Part model, mm, in its own coordinate system. Face numbers are marked on the shaded views. A direction names the side the tool comes from. Round coordinates to 2 decimals unless told otherwise and drop trailing zeros. Loops run counter-clockwise (first coordinate to the right, second up) from the corner with the lowest first, then second, coordinate; pieces in that order, holes last. Notation, with made-up numbers: (16, -8.75) -> (30, -8.75) arc R11 ccw to (30, 9.25) -> close; hole circle Ø11 at (-9, 79). An arc over 180 degrees is marked (long way). Answer as CSV lines item,"result".
from build123d import *

# Parameters (mm, degrees)
EXTRUDE_THIN1_DEPTH        = 36
CONVERT_SOLID1_START       = -36
CONVERT_SOLID1_DEPTH       = 72
CONVERT_SOLID1_2_DEPTH     = 72
F_6_5_6_5_DIAMETER_HOLE1_D = 6.5
F_6_5_6_5_DIAMETER_HOLE2_D = 6.5


# Read off the part's stored shape, not the designer's step: Convert-Solid1
with BuildPart() as part:
    # Sketch1 → Extrude-Thin1 (new, symmetric)
    with BuildSketch(Plane.XY):
        Polygon((-50, -56), (-50, 0), (50, 0), (50, -56), (46, -56), (46, -4), (-46, -4), (-46, -56), align=None)
    extrude(amount=EXTRUDE_THIN1_DEPTH, both=True)

    # Convert-Solid1 outline → Convert-Solid1 (cut)
    with BuildSketch(Plane.XY.offset(CONVERT_SOLID1_START)):
        with BuildLine():
            Line((50, 0), (44, 0))
            ThreePointArc((44, 0), (48.242640687, -1.757359313), (50, -6))
            Line((50, -6), (50, 0))
        make_face()
        with BuildLine():
            ThreePointArc((-50, -6), (-48.242640687, -1.757359313), (-44, 0))
            Line((-44, 0), (-50, 0))
            Line((-50, 0), (-50, -6))
        make_face()
    extrude(amount=CONVERT_SOLID1_DEPTH, mode=Mode.SUBTRACT)

    # Convert-Solid1 2 outline → Convert-Solid1 2 (add)
    with BuildSketch(Plane.XY.offset(CONVERT_SOLID1_START)):
        with BuildLine():
            Line((46, -4), (44, -4))
            ThreePointArc((44, -4), (45.414213562, -4.585786438), (46, -6))
            Line((46, -6), (46, -4))
        make_face()
        with BuildLine():
            ThreePointArc((-46, -6), (-45.414213562, -4.585786438), (-44, -4))
            Line((-44, -4), (-46, -4))
            Line((-46, -4), (-46, -6))
        make_face()
    extrude(amount=CONVERT_SOLID1_2_DEPTH)

    # Ø6.5 (6.5) Diameter Hole1 (through all)
    with Locations(Plane(origin=(-92.5, 4, 244.5), x_dir=(1, 0, 0), z_dir=(0, 1, 0))):
        with Locations((-122.5, 244.5), (-62.5, 244.5), (62.5, 244.5), (122.5, 244.5)):
            Hole(F_6_5_6_5_DIAMETER_HOLE1_D / 2)

    # Ø6.5 (6.5) Diameter Hole2 (through all)
    with Locations(Plane(origin=(92.5, 4, 244.5), x_dir=(1, 0, 0), z_dir=(0, 1, 0))):
        with Locations((-122.5, 244.5), (-62.5, 244.5), (62.5, 244.5), (122.5, 244.5)):
            Hole(F_6_5_6_5_DIAMETER_HOLE2_D / 2)


solid = part.part
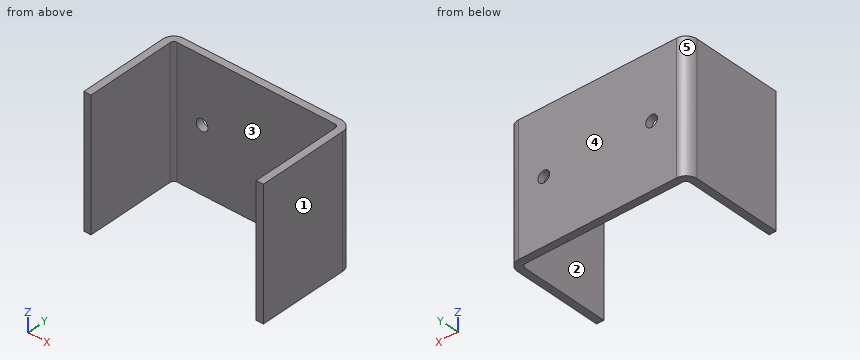
Q1. Saw through at B-B, the plane y = -41.5. Write the cut outline in (x, z), then the cut area to 3 significant figures.
Geometry results:
outline,"(-50, -36) -> (-46, -36) -> (-46, 36) -> (-50, 36) -> close; (46, -36) -> (50, -36) -> (50, 36) -> (46, 36) -> close"
area,"576 mm2"
Q2. Which spindle directions (+Z, -Z, +X, -X, +Y, -Y) get a long thin tool onto all of the face, cutting with end or side? Do the marked faces 1 and 2. Say none if no direction does.
Geometry results:
face 1,"+Z, -Z, +X, +Y, -Y"
face 2,"+Z, -Z, -Y"
Q3. Saw through at C-C, the plane z = 26. Write the cut outline in (x, y).
Geometry results:
outline,"(-50, -56) -> (-46, -56) -> (-46, -6) arc R2 cw to (-44, -4) -> (44, -4) arc R2 cw to (46, -6) -> (46, -56) -> (50, -56) -> (50, -6) arc R6 ccw to (44, 0) -> (-44, 0) arc R6 ccw to (-50, -6) -> close"
Q4. Saw through at A-A, the plane x = -30. Write the cut outline in (y, z), then the cut area to 3 significant figures.
Geometry results:
outline,"(-4, -36) -> (0, -36) -> (0, -3.25) -> (-4, -3.25) -> close; (-4, 3.25) -> (0, 3.25) -> (0, 36) -> (-4, 36) -> close"
area,"262 mm2"
Q5. Drill centre lines: line 1 along X through (y, z) = (-40, -24.5); line 2 along Z through (x, y) = (30, -3.15); line 3 along Y through (x, z) = (-22.5, -17). Where is each one in solid material? Low to high.
Geometry results:
line 1,"-50 to -46, 46 to 50"
line 2,"-36 to -3.25, 3.25 to 36"
line 3,"-4 to 0"
Q6. Drop flat-ended pins along their axis: P1, Ø21.5, axis at x = -20, z = -5.5, coming from the -Y side; P2, Ø6, axis at x = 30, z = 0, coming from the +Y side. Give the stop position or say it passes through.
Geometry results:
P1,"y = -4"
P2,"through"
Q7. Two-plate mould, pull along X, no slides. Class the marked faces 3, 4 and 5: pulls with the +X half, pulls with the -X half, needs draft (parallel to the pull), parting line crosses it, or undercut.
Geometry results:
face 3,"undercut"
face 4,"needs draft"
face 5,"pulls with the -X half"
Q8. Saw through at D-D, the plane z = 0. Write the cut outline in (x, y), then the cut area to 3 significant figures.
Geometry results:
outline,"(-50, -56) -> (-46, -56) -> (-46, -6) arc R2 cw to (-44, -4) -> (-33.25, -4) -> (-33.25, 0) -> (-44, 0) arc R6 ccw to (-50, -6) -> close; (-26.75, -4) -> (26.75, -4) -> (26.75, 0) -> (-26.75, 0) -> close; (33.25, -4) -> (44, -4) arc R2 cw to (46, -6) -> (46, -56) -> (50, -56) -> (50, -6) arc R6 ccw to (44, 0) -> (33.25, 0) -> close"
area,"750 mm2"
